from build123d import *

# Parameters (mm, degrees)
BOSS_EXTRUDE1_DEPTH = 6.35
SKETCH3_R           = 1.1303
SKETCH3_W           = 10.16
SKETCH3_H           = 15.24
CUT_EXTRUDE1_DEPTH  = 6.35
SKETCH5_W           = 28.194
SKETCH5_H           = 95.25
CUT_EXTRUDE2_DEPTH  = 6.35
SKETCH6_W           = 13.337799598
SKETCH6_H           = 13.337799598
CUT_EXTRUDE3_DEPTH  = 6.35
SKETCH7_R           = 1.1303
CUT_EXTRUDE4_DEPTH  = 16.002
SKETCH8_R           = 1.1303
SKETCH8_W           = 10.16
SKETCH8_H           = 15.24
CUT_EXTRUDE5_DEPTH  = 6.35
SKETCH9_W           = 12.065
SKETCH9_H           = 6.35
SKETCH9_W_2         = 12.192
BOSS_EXTRUDE2_DEPTH = 3.175
SKETCH10_W          = 12.192
SKETCH10_H          = 6.35
SKETCH10_W_2        = 12.065
BOSS_EXTRUDE3_DEPTH = 3.175
SKETCH12_R          = 1.1303
CUT_EXTRUDE7_DEPTH  = 19.05
SKETCH14_R          = 1.1303
CUT_EXTRUDE8_DEPTH  = 6.35
SKETCH15_R          = 1.1303
CUT_EXTRUDE9_DEPTH  = 6.35


with BuildPart() as part:
    # Sketch1 → Boss-Extrude1 (new body)
    with BuildSketch(Plane(origin=(0, 0, 0), x_dir=(1, 0, 0), z_dir=(0, 1, 0))):
        Polygon((0, 0), (60.96, 0), (60.96, 116.332), (205.74, 116.332), (205.74, 0), (266.7, 0), (266.7, 266.7), (0, 266.7), align=None)
    extrude(amount=BOSS_EXTRUDE1_DEPTH)

    # Sketch3 → Cut-Extrude1 (cut)
    with BuildSketch(Plane.XZ):
        with Locations(Location((38.2651, -232.41, 0), (0, 0, 270))):
            Circle(SKETCH3_R)
        with Locations(Location((38.2651, -207.01, 0), (0, 0, 270))):
            Circle(SKETCH3_R)
        with Locations(Location((76.0857, -223.012, 0), (0, 0, 270))):
            Circle(SKETCH3_R)
        with Locations(Location((76.0857, -200.66, 0), (0, 0, 270))):
            Circle(SKETCH3_R)
        with Locations(Location((107.8611, -166.37, 0), (0, 0, 270))):
            Circle(SKETCH3_R)
        with Locations(Location((107.8611, -196.85, 0), (0, 0, 270))):
            Circle(SKETCH3_R)
        with Locations(Location((129.4511, -166.37, 0), (0, 0, 270))):
            Circle(SKETCH3_R)
        with Locations(Location((129.4511, -196.85, 0), (0, 0, 270))):
            Circle(SKETCH3_R)
        with Locations(Location((137.2743, -217.17, 0), (0, 0, 270))):
            Circle(SKETCH3_R)
        with Locations(Location((158.8643, -217.17, 0), (0, 0, 270))):
            Circle(SKETCH3_R)
        with Locations(Location((137.2743, -247.65, 0), (0, 0, 270))):
            Circle(SKETCH3_R)
        with Locations(Location((158.8643, -247.65, 0), (0, 0, 270))):
            Circle(SKETCH3_R)
        with Locations(Location((190.5889, -191.008, 0), (0, 0, 270))):
            Circle(SKETCH3_R)
        with Locations(Location((190.5889, -213.36, 0), (0, 0, 270))):
            Circle(SKETCH3_R)
        with Locations(Location((228.4349, -181.61, 0), (0, 0, 270))):
            Circle(SKETCH3_R)
        with Locations(Location((228.4349, -207.01, 0), (0, 0, 270))):
            Circle(SKETCH3_R)
        with Locations((205.3209, -207.01)):
            Rectangle(SKETCH3_W, SKETCH3_H)
        with Locations((61.3537, -207.01)):
            Rectangle(SKETCH3_W, SKETCH3_H)
    extrude(amount=-CUT_EXTRUDE1_DEPTH, mode=Mode.SUBTRACT)

    # Sketch5 → Cut-Extrude2 (cut)
    with BuildSketch(Plane(origin=(0, 0, 0), x_dir=(1, 0, 0), z_dir=(0, 1, 0))):
        with Locations((14.097, 207.01)):
            Rectangle(SKETCH5_W, SKETCH5_H)
        with Locations((252.603, 207.01)):
            Rectangle(SKETCH5_W, SKETCH5_H)
        with Locations((252.603, 59.817)):
            Rectangle(SKETCH5_W, SKETCH5_H)
        with Locations((14.097, 59.817)):
            Rectangle(SKETCH5_W, SKETCH5_H)
    extrude(amount=CUT_EXTRUDE2_DEPTH, mode=Mode.SUBTRACT)

    # Sketch6 → Cut-Extrude3 (cut)
    with BuildSketch(Plane(origin=(0, 6.35, 0), x_dir=(1, 0, 0), z_dir=(0, 1, 0))):
        with Locations((73.102599799, 181.61)):
            Rectangle(SKETCH6_W, SKETCH6_H)
        with Locations((193.572000201, 232.41)):
            Rectangle(SKETCH6_W, SKETCH6_H)
    extrude(amount=-CUT_EXTRUDE3_DEPTH, mode=Mode.SUBTRACT)

    # Sketch7 → Cut-Extrude4 (cut)
    with BuildSketch(Plane.XZ):
        with Locations(Location((38.2651, -34.29, 0), (0, 0, 270))):
            Circle(SKETCH7_R)
        with Locations(Location((38.2651, -59.69, 0), (0, 0, 270))):
            Circle(SKETCH7_R)
        with Locations(Location((228.4349, -34.29, 0), (0, 0, 270))):
            Circle(SKETCH7_R)
        with Locations(Location((228.4349, -59.69, 0), (0, 0, 270))):
            Circle(SKETCH7_R)
    extrude(amount=-CUT_EXTRUDE4_DEPTH, mode=Mode.SUBTRACT)

    # Sketch8 → Cut-Extrude5 (cut)
    with BuildSketch(Plane(origin=(0, 6.35, 0), x_dir=(1, 0, 0), z_dir=(0, 1, 0))):
        with Locations(Location((14.859, 146.1135, 0), (0, 0, 270))):
            Circle(SKETCH8_R)
        with Locations(Location((14.859, 120.7135, 0), (0, 0, 270))):
            Circle(SKETCH8_R)
        with Locations(Location((54.229, 146.1135, 0), (0, 0, 270))):
            Circle(SKETCH8_R)
        with Locations(Location((54.229, 120.7135, 0), (0, 0, 270))):
            Circle(SKETCH8_R)
        with Locations(Location((212.471, 146.1135, 0), (0, 0, 270))):
            Circle(SKETCH8_R)
        with Locations(Location((212.471, 120.7135, 0), (0, 0, 270))):
            Circle(SKETCH8_R)
        with Locations(Location((251.841, 120.7135, 0), (0, 0, 270))):
            Circle(SKETCH8_R)
        with Locations(Location((251.841, 146.1135, 0), (0, 0, 270))):
            Circle(SKETCH8_R)
        with Locations(Location((139.065, 154.432, 0), (0, 0, 270))):
            Circle(SKETCH8_R)
        with Locations(Location((139.065, 129.032, 0), (0, 0, 270))):
            Circle(SKETCH8_R)
        with Locations(Location((176.911, 160.782, 0), (0, 0, 270))):
            Circle(SKETCH8_R)
        with Locations(Location((176.911, 138.43, 0), (0, 0, 270))):
            Circle(SKETCH8_R)
        with Locations(Location((238.125, 144.272, 0), (0, 0, 270))):
            Circle(SKETCH8_R)
        with Locations(Location((238.125, 113.792, 0), (0, 0, 270))):
            Circle(SKETCH8_R)
        with Locations(Location((259.715, 144.272, 0), (0, 0, 270))):
            Circle(SKETCH8_R)
        with Locations(Location((259.715, 113.792, 0), (0, 0, 270))):
            Circle(SKETCH8_R)
        with Locations((160.782, 154.432)):
            Rectangle(SKETCH8_W, SKETCH8_H)
    extrude(amount=-CUT_EXTRUDE5_DEPTH, mode=Mode.SUBTRACT)

    # Sketch9 → Boss-Extrude2 (add)
    with BuildSketch(Plane.ZY):
        with Locations((-260.6675, 3.175)):
            Rectangle(SKETCH9_W, SKETCH9_H)
        with Locations((-6.096, 3.175)):
            Rectangle(SKETCH9_W_2, SKETCH9_H)
        with Locations((-153.289, 3.175)):
            Rectangle(SKETCH9_W_2, SKETCH9_H)
        with Locations((-113.538, 3.175)):
            Rectangle(SKETCH9_W_2, SKETCH9_H)
    extrude(amount=BOSS_EXTRUDE2_DEPTH)

    # Sketch10 → Boss-Extrude3 (add)
    with BuildSketch(Plane(origin=(266.7, 0, 0), x_dir=(0, 0, -1), z_dir=(1, 0, 0))):
        with Locations((6.096, 3.175)):
            Rectangle(SKETCH10_W, SKETCH10_H)
        with Locations((113.538, 3.175)):
            Rectangle(SKETCH10_W, SKETCH10_H)
        with Locations((153.289, 3.175)):
            Rectangle(SKETCH10_W, SKETCH10_H)
        with Locations((260.6675, 3.175)):
            Rectangle(SKETCH10_W_2, SKETCH10_H)
    extrude(amount=BOSS_EXTRUDE3_DEPTH)

    # Sketch12 → Cut-Extrude7 (cut)
    with BuildSketch(Plane(origin=(0, 6.35, 0), x_dir=(1, 0, 0), z_dir=(0, 1, 0))):
        with Locations(Location((100.965, 219.71, 0), (0, 0, 270))):
            Circle(SKETCH12_R)
        with Locations(Location((100.965, 194.31, 0), (0, 0, 270))):
            Circle(SKETCH12_R)
        with Locations(Location((165.735, 219.71, 0), (0, 0, 270))):
            Circle(SKETCH12_R)
        with Locations(Location((165.735, 194.31, 0), (0, 0, 270))):
            Circle(SKETCH12_R)
    extrude(amount=-CUT_EXTRUDE7_DEPTH, mode=Mode.SUBTRACT)

    # Sketch14 → Cut-Extrude8 (cut)
    with BuildSketch(Plane.XZ):
        with Locations(Location((6.477, -133.985, 0), (0, 0, 270))):
            Circle(SKETCH14_R)
        with Locations(Location((6.477, -112.522, 0), (0, 0, 270))):
            Circle(SKETCH14_R)
        with Locations(Location((260.223, -132.842, 0), (0, 0, 270))):
            Circle(SKETCH14_R)
        with Locations(Location((260.223, -154.305, 0), (0, 0, 270))):
            Circle(SKETCH14_R)
    extrude(amount=-CUT_EXTRUDE8_DEPTH, mode=Mode.SUBTRACT)

    # Sketch15 → Cut-Extrude9 (cut)
    with BuildSketch(Plane.XZ):
        with Locations(Location((6.477, -6.096, 0), (0, 0, 270))):
            Circle(SKETCH15_R)
        with Locations(Location((6.477, -260.722358198, 0), (0, 0, 270))):
            Circle(SKETCH15_R)
        with Locations(Location((260.223, -260.604, 0), (0, 0, 270))):
            Circle(SKETCH15_R)
        with Locations(Location((260.223, -6.096, 0), (0, 0, 270))):
            Circle(SKETCH15_R)
    extrude(amount=-CUT_EXTRUDE9_DEPTH, mode=Mode.SUBTRACT)


solid = part.part
CAD build for the part. Positions are in the model's coordinates, mm. A direction names the side the tool comes from. Coordinates: 2 decimals unless noted, no trailing zeros. Order: outer loops, then holes, each group sorted by start corner. A loop starts at its lowest first (then second) coordinate and runs counter-clockwise, first axis right, second up.
Item 1: Drill centre lines: L1, parallel to X at y = 2, z = -208.5; L2, parallel to Z at x = 137, y = 1.75; L3, parallel to X at y = 3.5, z = -219.71. Where is each one in solid material? Low to high.
Check sheet entries:
L1: x = 28.19 to 56.27, 66.43 to 200.24, 210.4 to 238.51
L2: z = -266.7 to -248.75, -246.55 to -218.27, -216.07 to -116.33
L3: x = 28.19 to 99.83, 102.1 to 164.6, 166.87 to 238.51
Item 2: Band-saw the part on A-A on z = -45.5. List the corners of the cut face in (x, y), plus the area to 3 significant figures.
Check sheet entries:
outline: (28.19, 0) - (60.96, 0) - (60.96, 6.35) - (28.19, 6.35) - close; (205.74, 0) - (238.51, 0) - (238.51, 6.35) - (205.74, 6.35) - close
area: 416 mm2
Item 3: Band-saw the part on C-C on y = 3.5. Give the number of separate pieces and of enclosed holes in the cut face, plus the area to 3 significant figures.
Check sheet entries:
separate pieces: 1
enclosed holes: 53
area: 42,800 mm2
Item 4: Pin check, flat tips, straight feed: pin 1 Ø3 at (y, z) = (4.5, -139) entering from -X; pin 2 Ø1.9 at (y, z) = (3.5, -232.5) entering from -X; pin 3 Ø2 at (x, z) = (100.965, -219.71) entering from +Y; pin 4 Ø1.9 at (y, z) = (2, -218) entering from +X. Stop position of each tip, or through.
Check sheet entries:
pin 1: stops at x = 0
pin 2: stops at x = 28.19
pin 3: passes through
pin 4: stops at x = 238.51
Item 5: 3-axis set-ups, long thin cutter, end or side, ignore diameter. For faces 1 (the face through (193, 3, -225.741)), 2 (the face through (254, 3, -107.442)), 3 (the face through (13, 3, -254.635)), 4 (the face through (269.875, 3, -6)): which of +Z, -Z, +X, -X, +Y, -Y reach the whole face in a straight line?
Check sheet entries:
face 1: +Y, -Y
face 2: +X, +Y, -Y
face 3: -X, +Y, -Y
face 4: +Z, -Z, +X, +Y, -Y
Item 6: Band-saw the part on B-B on x = 120. List the corners of the cut face in (y, z).
Check sheet entries:
outline: (0, -266.7) - (6.35, -266.7) - (6.35, -116.33) - (0, -116.33) - close
